Study the drawing (mm; zero at the part's minimum x, y, z) and answer. A direction names the side the tool comes from. Coordinates: 2 decimals unless noted, no trailing zeros. Loops run counter-clockwise (first coordinate to the right, second up) from the corner with the lowest first, then second, coordinate; pieces in that order, holes last. Notation, with made-up numbers: (23.25, 4.25) - (81.25, 4.25) arc R11 cw to (81.25, 23.25) - close; hole circle Ø9 at (21, 64). An arc over 180 degrees is marked (long way). Put each result on its own line as item: value.
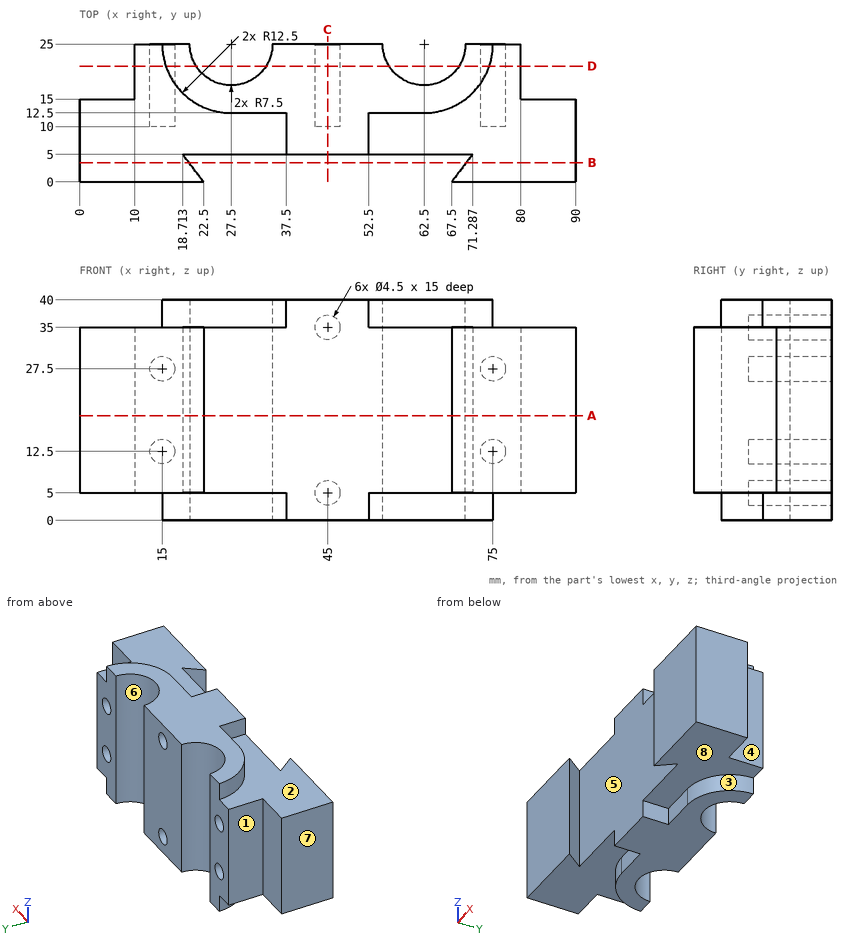
1) Straight lines are drawn through the part: L1, parallel to Z at x = 45, y = 22.25; L2, parallel to Z at x = 75, y = 19.5; L3, parallel to X at y = 20.75, z = 21. For each, find the intervals that lie inside material, in ascending order. Write a range as [from, to].
Found:
L1: z = [0, 2.75], [7.25, 32.75], [37.25, 40]
L2: z = [5, 10.25], [14.75, 25.25], [29.75, 35]
L3: x = [10, 21.32], [33.68, 56.32], [68.68, 80]
2) For a pull along X with two mould halves and no side action, classify the marked faces 5, 6, 7 and 8 as pulls with the +X half, pulls with the -X half, needs draft (parallel to the pull), parting line crosses it, or undercut.
Found:
face 5: undercut
face 6: undercut
face 7: pulls with the -X half
face 8: needs draft
3) For the marked faces 1, 2, 3 and 4, determine the directions among +Z, -Z, +X, -X, +Y, -Y from which every point of the face is accessible in a straight line to the end or side of a thin tool.
Found:
face 1: +Z, -Z, -X, +Y
face 2: +Z, -X, -Y
face 3: -Z, +X, -Y
face 4: +Z, -Z, +X, +Y
4) Each of these flat-tipped pins is pushed along its axis until it touches: pin 1 (5 mm diameter, centred on x = 45, z = 5, fed in from -Y); pin 2 (3 mm diameter, centred on x = 18.5, z = 22, fed in from -Y); pin 3 (2 mm diameter, centred on x = 75, z = 28, fed in from +Y); pin 4 (5 mm diameter, centred on y = 19, z = 19, fed in from -X). Where does it stop, or does it pass through?
Found:
pin 1: stops at y = 5
pin 2: stops at y = 0
pin 3: stops at y = 10
pin 4: stops at x = 10
5) The part is cut by section B-B (y = 3.5). Give the vertices of the cut face in (x, z).
Found:
outline: (0, 5) - (19.85, 5) - (19.85, 35) - (0, 35) - close; (70.15, 5) - (90, 5) - (90, 35) - (70.15, 35) - close
6) The part is cut by section C-C (x = 45). Give the vertices of the cut face in (y, z), and give its area (3 significant figures).
Found:
outline: (5, 0) - (25, 0) - (25, 2.75) - (10, 2.75) - (10, 7.25) - (25, 7.25) - (25, 32.75) - (10, 32.75) - (10, 37.25) - (25, 37.25) - (25, 40) - (5, 40) - close
area: 665 mm^2
7) The part is cut by section A-A (z = 19). Give the vertices of the cut face in (x, y), and give its area (3 significant figures).
Found:
outline: (0, 0) - (22.5, 0) - (18.71, 5) - (71.29, 5) - (67.5, 0) - (90, 0) - (90, 15) - (80, 15) - (80, 25) - (70, 25) arc R7.5 cw to (55, 25) - (35, 25) arc R7.5 cw to (20, 25) - (10, 25) - (10, 15) - (0, 15) - close
area: 1,630 mm^2
8) The part is cut by section D-D (y = 21). State how many separate pieces and enclosed holes the cut face has, and give its area (3 significant figures).
Found:
separate pieces: 3
enclosed holes: 6
area: 1,580 mm^2
